For this review, take the finished solid that the model builds, in its own axes (mm). A direction names the side the tool comes from. Give positions to 0.01 mm unless a question says otherwise; leave off trailing zeros. Order: outer loops, then holes, each group sorted by start corner. A loop starts at its lowest first (then second) coordinate and runs counter-clockwise, first axis right, second up. Notation, with made-up numbers: (83.5, 75) - (110.5, 75) arc R25 cw to (110.5, 108) - close; hole circle Ø4 at (37, 72). An arc over 180 degrees is marked (long way). Use a Markdown table: item, result. Add a question column.
1) Mouldability with a two-part tool opening along Y and no side actions: class faces 4 (the face through (-5.711, -10.614, 9.043)), 5 (the face through (-12.88, 11.81, 5.42)), 6 (the face through (-8, 0, 0)) as released by +Y, released by -Y, zero draft, split by the parting line, or undercut.
2) We need section D-D on y = 7. Write out the cut boundary in (x, z), then the cut area to 3 significant figures.
3) Machinability: for faces 1 (the face through (-14.1, 0.09, 4.06)), 2 (the face through (0, 14, 8)), 3 (the face through (5.158, -3.955, 3.204)), which of the approach directions +Z, -Z, +X, -X, +Y, -Y give a long, thin tool a straight path to every point of the face, cutting with its end or side? Answer none if there is none.
4) We need section C-C on x = -1. Write out the cut boundary in (y, z), then the cut area to 3 significant figures.
5) Wall thickness on L1, parallel to Y at x = 0, z = 9.05 (3 decimals); L2, parallel to X at y = -1, z = 7; L3, parallel to X at y = -9.5, z = 5.75: over which ranges is each line inside the solid? List them lowest first.
6) We need section B-B on y = -4.5. Write out the cut boundary in (x, z).
7) We need section A-A on z = 10. Write out the cut boundary in (x, y) (3 decimals).
8) Clearance check with flat-ended pins moving along their axes: P1, Ø1.9, axis at x = 0, y = -14, coming from the +Z side; P2, Ø11.5, axis at x = 0, y = 0, coming from the -Z side. State where each tip first meets the part, or that it passes through.
```python
from build123d import *

# Parameters (mm, degrees)
SKETCH1_R             = 17.475
SKETCH1_R_2           = 8.025
BOSS_EXTRUDE1_DEPTH   = 12
CUT_EXTRUDE1_START    = 12
SKETCH1_3_R           = 1.55
CUT_EXTRUDE1_DEPTH    = 4
BOSS_EXTRUDE2_START   = 11
SKETCH1_4_R           = 18.5
SKETCH1_4_R_2         = 17.475
BOSS_EXTRUDE2_DEPTH   = 1
SKETCH2_R             = 8.025
SKETCH2_R_2           = 6.5
BOSS_EXTRUDE3_DEPTH   = 12
CUT_EXTRUDE2_START    = -6.5
SKETCH2_2_R           = 8.025
SKETCH2_2_R_2         = 6.5
CUT_EXTRUDE2_DEPTH    = 5.5
M5_TAPPED_HOLE1_D     = 4.2
M5_TAPPED_HOLE1_DEPTH = 8
M5_TAPPED_HOLE1_TIP   = 1.2618073


with BuildPart() as part:
    # Sketch1 → Boss-Extrude1 (new body)
    with BuildSketch(Plane.XY):
        Circle(SKETCH1_R)
        Circle(SKETCH1_R_2, mode=Mode.SUBTRACT)
    extrude(amount=BOSS_EXTRUDE1_DEPTH)

    # Sketch1<3> → Cut-Extrude1 (cut)
    with BuildSketch(Plane.XY.offset(CUT_EXTRUDE1_START)):
        with Locations((-12.124355653, 7)):
            Circle(SKETCH1_3_R)
        with BuildLine():
            ThreePointArc((0, 15.55), (-1.55, 14), (0, 12.45))
            Line((0, 12.45), (0, 15.55))
        make_face()
        with BuildLine():
            Line((0, 15.55), (0, 12.45))
            ThreePointArc((0, 12.45), (1.096015511, 12.903984489), (1.55, 14))
            ThreePointArc((1.55, 14), (1.096015511, 15.096015511), (0, 15.55))
        make_face()
        with Locations((12.124355653, 7)):
            Circle(SKETCH1_3_R)
        with Locations((12.124355653, -7)):
            Circle(SKETCH1_3_R)
        with Locations((0, -14)):
            Circle(SKETCH1_3_R)
        with Locations((-12.124355653, -7)):
            Circle(SKETCH1_3_R)
    extrude(amount=-CUT_EXTRUDE1_DEPTH, mode=Mode.SUBTRACT)

    # Sketch1<4> → Boss-Extrude2 (add)
    with BuildSketch(Plane.XY.offset(BOSS_EXTRUDE2_START)):
        Circle(SKETCH1_4_R)
        Circle(SKETCH1_4_R_2, mode=Mode.SUBTRACT)
    extrude(amount=BOSS_EXTRUDE2_DEPTH)

    # Sketch2 → Boss-Extrude3 (add)
    with BuildSketch(Plane(origin=(0, 0, 0), x_dir=(-1, 0, 0), z_dir=(0, 0, -1))):
        Circle(SKETCH2_R)
        Circle(SKETCH2_R_2, mode=Mode.SUBTRACT)
    extrude(amount=-BOSS_EXTRUDE3_DEPTH)

    # Sketch2<2> → Cut-Extrude2 (cut)
    with BuildSketch(Plane(origin=(0, 0, 0), x_dir=(-1, 0, 0), z_dir=(0, 0, -1)).offset(CUT_EXTRUDE2_START)):
        with Locations(Location((0, 0, 0), (0, 0, 180))):
            Circle(SKETCH2_2_R)
        Circle(SKETCH2_2_R_2, mode=Mode.SUBTRACT)
    extrude(amount=-CUT_EXTRUDE2_DEPTH, mode=Mode.SUBTRACT)

    # M5 Tapped Hole1
    with Locations(Plane(origin=(0, 0, 0), x_dir=(-1, 0, 0), z_dir=(0, 0, -1))):
        with Locations((-12, 0), (-6, -10.392304845), (6, -10.392304845), (6, 10.392304845), (12, 0), (-6, 10.392304845)):
            Hole(M5_TAPPED_HOLE1_D / 2, depth=M5_TAPPED_HOLE1_DEPTH)
            with Locations((0, 0, -(M5_TAPPED_HOLE1_DEPTH + M5_TAPPED_HOLE1_TIP / 2))):  # 118° drill point
                Cone(0, M5_TAPPED_HOLE1_D / 2, M5_TAPPED_HOLE1_TIP, mode=Mode.SUBTRACT)


solid = part.part
```
Checked values:
| question | item | result |
|---|---|---|
| 1 | face 4 | undercut |
| 1 | face 5 | split by the parting line |
| 1 | face 6 | zero draft |
| 2 | outline | (-17.12, 11) - (-16.01, 11) - (-16.01, 0) - (16.01, 0) - (16.01, 11) - (17.12, 11) - (17.12, 12) - (13.67, 12) - (13.67, 8) - (10.57, 8) - (10.57, 12) - (3.92, 12) - (3.92, 6.5) - (-3.92, 6.5) - (-3.92, 12) - (-10.57, 12) - (-10.57, 8) - (-13.67, 8) - (-13.67, 12) - (-17.12, 12) - close |
| 2 | area | 319 mm² |
| 3 | face 1 | -Z |
| 3 | face 2 | +Z |
| 3 | face 3 | +Z, -Z |
| 4 | outline | (-18.47, 11) - (-17.45, 11) - (-17.45, 0) - (-6.42, 0) - (-6.42, 6.5) - (-7.96, 6.5) - (-7.96, 12) - (-12.82, 12) - (-12.82, 8) - (-15.18, 8) - (-15.18, 12) - (-18.47, 12) - close; (6.42, 0) - (17.45, 0) - (17.45, 11) - (18.47, 11) - (18.47, 12) - (15.18, 12) - (15.18, 8) - (12.82, 8) - (12.82, 12) - (7.96, 12) - (7.96, 6.5) - (6.42, 6.5) - close |
| 4 | area | 231 mm² |
| 5 | L1 | -17.475 to -15.55, -12.45 to -8.025, 8.025 to 12.45, 15.55 to 17.475 |
| 5 | L2 | -17.45 to -13.85, -10.15 to -7.96, 7.96 to 10.15, 13.85 to 17.45 |
| 5 | L3 | -14.67 to -7.9, -4.1 to 4.1, 7.9 to 14.67 |
| 6 | outline | (-17.94, 11) - (-16.89, 11) - (-16.89, 0) - (-4.69, 0) - (-4.69, 6.5) - (-6.64, 6.5) - (-6.64, 12) - (-17.94, 12) - close; (4.69, 0) - (16.89, 0) - (16.89, 11) - (17.94, 11) - (17.94, 12) - (6.64, 12) - (6.64, 6.5) - (4.69, 6.5) - close |
| 7 | outline | circle Ø34.95 at (0, 0); hole circle Ø3.1 at (-12.124, -7); hole circle Ø3.1 at (-12.124, 7); hole circle Ø16.05 at (0, 0); hole circle Ø3.1 at (0, -14); hole circle Ø3.1 at (0, 14); hole circle Ø3.1 at (12.124, -7); hole circle Ø3.1 at (12.124, 7) |
| 8 | P1 | z = 8 |
| 8 | P2 | through |
